For this review, take the finished solid that the model builds, in its own axes (mm). A direction names the side the tool comes from. Coordinates: 2 decimals unless noted, no trailing zeros. Order: outer loops, then holes, each group sorted by start corner. A loop starts at its lowest first (then second) coordinate and runs counter-clockwise, first axis right, second up.
from build123d import *

# Parameters (mm, degrees)
SKETCH1_W       = 24
SKETCH1_H       = 8
EXTRUDE1_DEPTH  = 3.3
SKETCH2_R       = 2.25
EXTRUDE2_DEPTH  = 2
SKETCH3_W       = 4.5
SKETCH3_H       = 4.5
EXTRUDE3_DEPTH  = 2.5
LPATTERN1_COUNT = 4
LPATTERN1_PITCH = 8
LPATTERN2_COUNT = 4
LPATTERN2_PITCH = 8


with BuildPart() as part:
    # Sketch1 → Extrude1 (new body)
    with BuildSketch(Plane(origin=(0, 0, 0), x_dir=(1, 0, 0), z_dir=(0, 1, 0))):
        with Locations((12, 4)):
            Rectangle(SKETCH1_W, SKETCH1_H)
    extrude(amount=EXTRUDE1_DEPTH)

    # Sketch2 → Extrude2 (add)
    with BuildSketch(Plane(origin=(0, 3.3, 0), x_dir=(1, 0, 0), z_dir=(0, 1, 0))):
        with Locations(Location((4, 4, 0), (0, 0, 90))):
            Circle(SKETCH2_R)
    extrude2 = extrude(amount=EXTRUDE2_DEPTH)

    # Sketch3 → Extrude3 (cut)
    with BuildSketch(Plane.XZ):
        with Locations((20, -4)):
            Rectangle(SKETCH3_W, SKETCH3_H)
    extrude3 = extrude(amount=-EXTRUDE3_DEPTH, mode=Mode.SUBTRACT)

    # LPattern1: Extrude2 ×4, 1 skipped
    with Locations(*[(i * LPATTERN1_PITCH, 0, 0) for i in range(1, LPATTERN1_COUNT) if i not in (3,)]):
        add(extrude2)

    # LPattern2: Extrude3 ×4
    with Locations(*[(-i * LPATTERN2_PITCH, 0, 0) for i in range(1, LPATTERN2_COUNT)]):
        add(extrude3, mode=Mode.SUBTRACT)


solid = part.part
1. Take a section at C-C, the plane z = -4. Give the boundary of the cut face in (x, y).
Answer below:
outline: (0, 0) - (1.75, 0) - (1.75, 2.5) - (6.25, 2.5) - (6.25, 0) - (9.75, 0) - (9.75, 2.5) - (14.25, 2.5) - (14.25, 0) - (17.75, 0) - (17.75, 2.5) - (22.25, 2.5) - (22.25, 0) - (24, 0) - (24, 3.3) - (22.25, 3.3) - (22.25, 5.3) - (17.75, 5.3) - (17.75, 3.3) - (14.25, 3.3) - (14.25, 5.3) - (9.75, 5.3) - (9.75, 3.3) - (6.25, 3.3) - (6.25, 5.3) - (1.75, 5.3) - (1.75, 3.3) - (0, 3.3) - close
2. The part is to be moulded in two halves that separate along X. For faces 4 (the face through (12, 1, -1.75)), 5 (the face through (0, 2, -4)), 6 (the face through (12, 2, -8)), say which applies: +X half, -X half, draft (parallel to the pull), parting line (faces both ways), or undercut.
Answer below:
face 4: undercut
face 5: -X half
face 6: draft
3. Take a section at D-D, the plane x = 4.5. Give the boundary of the cut face in (y, z), plus the area to 3 significant figures.
Answer below:
outline: (0, -8) - (3.3, -8) - (3.3, -6.19) - (5.3, -6.19) - (5.3, -1.81) - (3.3, -1.81) - (3.3, 0) - (0, 0) - (0, -1.75) - (2.5, -1.75) - (2.5, -6.25) - (0, -6.25) - close
area: 23.9 mm2
4. Take a section at B-B, the plane y = 4.8. Give the boundary of the cut face in (x, z).
Answer below:
outline: circle Ø4.5 at (4, -4); circle Ø4.5 at (12, -4); circle Ø4.5 at (20, -4)
5. Machinability: for faces 1 (the face through (24, 2, -4)), 2 (the face through (4, 1, -6.25)), 3 (the face through (22.196, 4.286, -3.512)), which of the approach directions +Z, -Z, +X, -X, +Y, -Y give a long, thin tool a straight path to every point of the face, cutting with its end or side? Answer none if there is none.
Answer below:
face 1: +Z, -Z, +X, +Y, -Y
face 2: -Y
face 3: +Y
6. Clearance check with flat-ended pins moving along their axes: pin 1 Ø1.3 at (x, z) = (20, -4.5) entering from -Y; pin 2 Ø1 at (x, y) = (18, 4.5) entering from +Z; pin 3 Ø2 at (y, z) = (4.5, -4) entering from +X. State where each tip first meets the part, or that it passes through.
Answer below:
pin 1: stops at y = 2.5
pin 2: stops at z = -2.32
pin 3: stops at x = 22.25
7. Take a section at A-A, the plane x = 20. Give the boundary of the cut face in (y, z).
Answer below:
outline: (0, -8) - (3.3, -8) - (3.3, -6.25) - (5.3, -6.25) - (5.3, -1.75) - (3.3, -1.75) - (3.3, 0) - (0, 0) - (0, -1.75) - (2.5, -1.75) - (2.5, -6.25) - (0, -6.25) - close
8. To check wall thickness, follow L1, parallel to X at y = 1.3, z = -5.75; L2, parallel to X at y = 4.35, z = -4; L3, parallel to Z at x = 11.25, y = 0.8. State the ranges of each line that lie inside material, in increasing order.
Answer below:
L1: x = 0 to 1.75, 6.25 to 9.75, 14.25 to 17.75, 22.25 to 24
L2: x = 1.75 to 6.25, 9.75 to 14.25, 17.75 to 22.25
L3: z = -8 to -6.25, -1.75 to 0
